from build123d import *

# Parameters (mm, degrees)
SKETCH_1_W          = 40
SKETCH_1_H          = 20
EXTRUDE_1_DEPTH     = 6
SKETCH_2_R          = 2.5
CUT_EXTRUDE_1_DEPTH = 24.151673806
EXTRUDE_START       = -15
EXTRUDE_2_OUTLINE_R = 11
EXTRUDE_2_DEPTH     = 15
EXTRUDE_START_2     = -8
SKETCH_6_R          = 11
SKETCH_6_R_2        = 5
EXTRUDE_3_DEPTH     = 8


# Read off the part's stored shape, not the designer's step: the extrude step
with BuildPart() as part:
    # Sketch 1 → Extrude 1 (new body)
    with BuildSketch(Plane.XY):
        Rectangle(SKETCH_1_W, SKETCH_1_H)
    extrude(amount=EXTRUDE_1_DEPTH)

    # Sketch 2 → Cut-Extrude 1 (cut, through all)
    with BuildSketch(Plane.XY.offset(6)):
        with Locations((10, 0)):
            Circle(SKETCH_2_R)
        with Locations((-1, 0)):
            Circle(SKETCH_2_R)
        with Locations((-12, 0)):
            Circle(SKETCH_2_R)
    extrude(amount=-CUT_EXTRUDE_1_DEPTH, mode=Mode.SUBTRACT)

    # Extrude 2 outline → Extrude 2 (add)
    with BuildSketch(Plane.XY.offset(6).offset(EXTRUDE_START)):
        with BuildLine():
            Line((20, 10), (20, 13.5))
            Line((20, 13.5), (-26.893967141, 13.5))
            Line((-26.893967141, 13.5), (-26.893967141, 13.384337644))
            ThreePointArc((-26.893967141, 13.384337644), (-45, 0), (-26.893967141, -13.384337644))
            Line((-26.893967141, -13.384337644), (-26.893967141, -13.5))
            Line((-26.893967141, -13.5), (20, -13.5))
            Line((20, -13.5), (20, -10))
            Line((20, -10), (-20, -10))
            Line((-20, -10), (-20, -8.660254038))
            ThreePointArc((-20, -8.660254038), (-17, 0), (-20, 8.660254038))
            Line((-20, 8.660254038), (-20, 10))
            Line((-20, 10), (20, 10))
        make_face()
        with Locations((-31, 0)):
            Circle(EXTRUDE_2_OUTLINE_R, mode=Mode.SUBTRACT)
    extrude(amount=EXTRUDE_2_DEPTH)

    # Sketch 6 → Extrude 3 (add)
    with BuildSketch(Plane.XY.offset(6).offset(EXTRUDE_START_2)):
        with Locations((-31, 0)):
            Circle(SKETCH_6_R)
        with Locations((-31, 0)):
            Circle(SKETCH_6_R_2, mode=Mode.SUBTRACT)
    extrude(amount=EXTRUDE_3_DEPTH)


solid = part.part
Model file for the job. Use its own axes, mm. A direction names the side the tool comes from. Coordinates: 2 decimals unless noted, no trailing zeros. Order: outer loops, then holes, each group sorted by start corner. A loop starts at its lowest first (then second) coordinate and runs counter-clockwise, first axis right, second up. Notation, with made-up numbers: (-26.5, 43) -> (-8.5, 43) arc R31 ccw to (-8.5, 76) -> close; hole circle Ø1 at (-18.75, -18.75). An arc over 180 degrees is marked (long way). Return JSON: item names as keys, results as strings. Group by question number.
Item 1: Saw through at A-A on y = 0. Write the cut outline in (x, z), then the cut area to 3 significant figures.
Item 2: Saw through at D-D on z = -2.75. Write the cut outline in (x, y), then the cut area to 3 significant figures.
Item 3: Tool access for faces 4 (the flat face through (-4, -13.5, -2)), 5 (the flat face through (-29, -5, -2)), 6 (the flat face through (0, 10, -5)): list every direction of +Z, -Z, +X, -X, +Y, -Y with a clear straight run to the whole face (end or side of a thin tool).
Item 4: Pull direction Y, two halves, no side cores. Call faces 1 (the flat face through (-3, 13.5, -2)), 2 (the flat face through (0, -10, -5)), 3 (the flat face through (-13, 3, 6)): pulls with the +Y half, pulls with the -Y half, needs draft (parallel to the pull), parting line crosses it, or undercut.
Item 5: Wall check: line 1 along Y through (x, z) = (-12, 1.7); line 2 along X through (y, z) = (-2.25, 2.75); line 3 along Y through (x, z) = (-31, -4). Give the ranges that are in metal, low to high. Write a range as [from, to].
Item 6: Flat gauge pins, fed straight in: P1, Ø8, axis at x = 7.5, z = 2, coming from the -Y side; P2, Ø1.5, axis at y = 9, z = -6.5, coming from the +X side; P3, Ø1, axis at x = -28.5, z = -6.5, coming from the +Y side. Where does each tip first touch, or does it go through?
Item 7: Saw through at C-C on z = 1.25. Write the cut outline in (x, y).
Item 8: Saw through at B-B on x = 10. Write the cut outline in (y, z), then the cut area to 3 significant figures.
Values found:
{
 "1": {"outline": "(-45, -9) -> (-42, -9) -> (-42, -2) -> (-36, -2) -> (-36, 6) -> (-45, 6) -> close; (-26, -2) -> (-20, -2) -> (-20, -9) -> (-17, -9) -> (-17, 0) -> (-14.5, 0) -> (-14.5, 6) -> (-26, 6) -> close; (-9.5, 0) -> (-3.5, 0) -> (-3.5, 6) -> (-9.5, 6) -> close; (1.5, 0) -> (7.5, 0) -> (7.5, 6) -> (1.5, 6) -> close; (12.5, 0) -> (20, 0) -> (20, 6) -> (12.5, 6) -> close", "area": "318 mm2"},
 "2": {"outline": "(-26.89, -13.5) -> (20, -13.5) -> (20, -10) -> (-20, -10) -> (-20, -8.66) arc R14 ccw to (-20, 8.66) -> (-20, 10) -> (20, 10) -> (20, 13.5) -> (-26.89, 13.5) -> (-26.89, 13.38) arc R14 ccw (long way) to (-26.89, -13.38) -> close; hole circle Ø22 at (-31, 0)", "area": "543 mm2"},
 "3": {"face 4": "+Z, -Z, +X, -Y", "face 5": "-Z", "face 6": "-Z, +X"},
 "4": {"face 1": "pulls with the +Y half", "face 2": "undercut", "face 3": "needs draft"},
 "5": {"line 1": "y = [-13.5, -2.5], [2.5, 13.5]", "line 2": "x = [-44.82, -35.47], [-26.53, -13.09], [-10.91, -2.09], [0.09, 8.91], [11.09, 20]", "line 3": "y = [-14, -11], [11, 14]"},
 "6": {"P1": "stops at y = -13.5", "P2": "stops at x = -19.69", "P3": "stops at y = 13.86"},
 "7": {"outline": "(-26.89, -13.5) -> (20, -13.5) -> (20, 13.5) -> (-26.89, 13.5) -> (-26.89, 13.38) arc R14 ccw (long way) to (-26.89, -13.38) -> close; hole circle Ø10 at (-31, 0); hole circle Ø5 at (-12, 0); hole circle Ø5 at (-1, 0); hole circle Ø5 at (10, 0)"},
 "8": {"outline": "(-13.5, -9) -> (-10, -9) -> (-10, 0) -> (-2.5, 0) -> (-2.5, 6) -> (-13.5, 6) -> close; (2.5, 0) -> (10, 0) -> (10, -9) -> (13.5, -9) -> (13.5, 6) -> (2.5, 6) -> close", "area": "195 mm2"}
}
